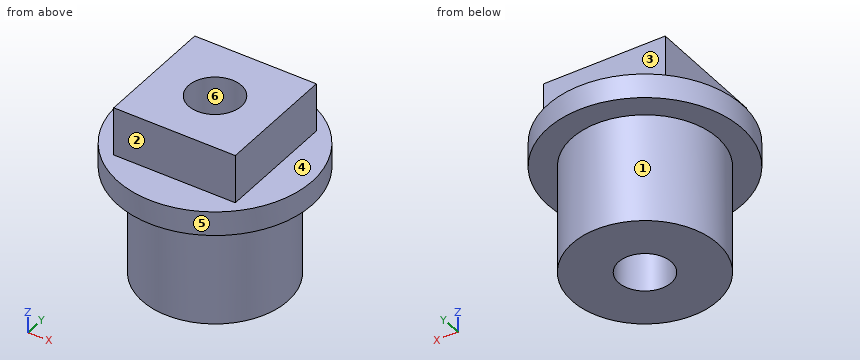
```python
from build123d import *

# Parameters (mm, degrees)
F0_R     = 4.7625
F0_R_2   = 1.7272
F1_DEPTH = 7.112
F2_R     = 6.35
F2_R_2   = 1.7272
F3_DEPTH = 1.5875
F4_W     = 7.9375
F4_H     = 7.9375
F4_R     = 1.7272
F5_DEPTH = 3.175


with BuildPart() as f1:
    # F0 (on Top) → F1 (new body)
    with BuildSketch(Plane.XY):
        Circle(F0_R)
        Circle(F0_R_2, mode=Mode.SUBTRACT)
    extrude(amount=F1_DEPTH)

    # F2 (on face) → F3 (join)
    with BuildSketch(Plane.XY.offset(7.112)):
        Circle(F2_R)
        Circle(F2_R_2, mode=Mode.SUBTRACT)
    extrude(amount=F3_DEPTH)

    # F4 (on face) → F5 (join)
    with BuildSketch(Plane.XY.offset(8.6995)):
        Rectangle(F4_W, F4_H)
        Circle(F4_R, mode=Mode.SUBTRACT)
    extrude(amount=F5_DEPTH)


solid = f1.part
```
The listing builds one solid part. Answer for the finished solid, in the listing's coordinates (mm). Face numbers are marked on the shaded views. A direction names the side the tool comes from. Give positions to 0.01 mm unless a question says otherwise; leave off trailing zeros. Order: outer loops, then holes, each group sorted by start corner. A loop starts at its lowest first (then second) coordinate and runs counter-clockwise, first axis right, second up. Notation, with made-up numbers: (28, -9.5) -> (39, -9.5) arc R23 ccw to (39, 4.5) -> close; hole circle Ø10 at (-2.75, 15). An arc over 180 degrees is marked (long way). Answer as a JSON object with one key per item and string values. Group by question number.
Item 1: The part is cut by section C-C on z = 10. Write down the section's boundary in (x, y).
Item 2: Determine the mould class of the marked faces 4, 5 and 6 for opening direction X: pulls with the +X half, pulls with the -X half, needs draft (parallel to the pull), parting line crosses it, or undercut.
Item 3: Consider L1, parallel to Y at x = 0, z = 8.75; L2, parallel to Y at x = 0, z = 5.5; L3, parallel to Y at x = 3.5, z = 10.25. Determine where each line is inside the solid, lowest interval first. Write a range as from..to.
Item 4: The part is cut by section D-D on y = -4.5. Write down the section's boundary in (x, z), and give its area (3 significant figures).
Item 5: Flat-ended cylindrical pins translate along their axes: pin 1 (2 mm diameter, centred on y = -5, z = 4, fed in from -X); pin 2 (2.5 mm diameter, centred on x = 2, z = 10, fed in from +Y); pin 3 (3 mm diameter, centred on x = -3.5, z = 3.5, fed in from -Y); pin 4 (3 mm diameter, centred on x = 0, y = 0, fed in from +Z). Find the tip coordinate at first contact, or state that the pin passes through.
Item 6: The part is cut by section A-A on y = 0. Write down the section's boundary in (x, z).
Item 7: A tool of negligible diameter and unlimited length cuts with its end or side. For the marked faces 1, 2 and 3, from which of +Z, -Z, +X, -X, +Y, -Y can it reach the whole face along a straight path? Write none if from no direction.
Result set:
{
 "1": {"outline": "(-3.97, -3.97) -> (3.97, -3.97) -> (3.97, 3.97) -> (-3.97, 3.97) -> close; hole circle Ø3.45 at (0, 0)"},
 "2": {"face 4": "needs draft", "face 5": "parting line crosses it", "face 6": "undercut"},
 "3": {"L1": "-3.97..-1.73, 1.73..3.97", "L2": "-4.76..-1.73, 1.73..4.76", "L3": "-3.97..3.97"},
 "4": {"outline": "(-4.48, 7.11) -> (-1.56, 7.11) -> (-1.56, 0) -> (1.56, 0) -> (1.56, 7.11) -> (4.48, 7.11) -> (4.48, 8.7) -> (-4.48, 8.7) -> close", "area": "36.4 mm²"},
 "5": {"pin 1": "x = -2.58", "pin 2": "y = 3.97", "pin 3": "y = -4.32", "pin 4": "through"},
 "6": {"outline": "(-6.35, 7.11) -> (-4.76, 7.11) -> (-4.76, 0) -> (-1.73, 0) -> (-1.73, 11.87) -> (-3.97, 11.87) -> (-3.97, 8.7) -> (-6.35, 8.7) -> close; (1.73, 0) -> (4.76, 0) -> (4.76, 7.11) -> (6.35, 7.11) -> (6.35, 8.7) -> (3.97, 8.7) -> (3.97, 11.87) -> (1.73, 11.87) -> close"},
 "7": {"face 1": "-Z", "face 2": "+Z, +X, -X, -Y", "face 3": "+Z, +X, -X, +Y"}
}
